Build history of the part. All positions in model axes, mm. A direction names the side the tool comes from. Coordinates: 2 decimals unless noted, no trailing zeros. Order: outer loops, then holes, each group sorted by start corner. A loop starts at its lowest first (then second) coordinate and runs counter-clockwise, first axis right, second up. Notation, with made-up numbers: (72.5, 27) - (122.5, 27) arc R36 ccw to (122.5, 66) - close; hole circle Ø4 at (50, 35). An arc over 180 degrees is marked (long way). Return JSON: item names as keys, results as strings.
from build123d import *

# Parameters (mm, degrees)
F1_DEPTH = 59.69
F2_DEPTH = 25.4
F4_DEPTH = 7.9375
F6_R     = 6.35


# Not quite as in the source:
# - a feature of the source that left no trace in its solid (it failed there, or was rolled back) is left out


with BuildPart() as f1:
    # F0 (on Front) → F1 (new body, symmetric)
    with BuildSketch(Plane.XZ):
        Polygon((22.225, 9.525), (-41.275, 9.525), (-41.275, -9.525), (41.275, -9.525), (41.275, 9.525), align=None)
    extrude(amount=F1_DEPTH, both=True)

    # F0 (on Front) → F2 (join, symmetric)
    with BuildSketch(Plane.XZ):
        with BuildLine():
            Line((22.225, 27.0002), (22.225, 9.525))
            Line((22.225, 9.525), (41.275, 9.525))
            Line((41.275, 9.525), (41.275, 27.0002))
            ThreePointArc((41.275, 27.0002), (45.9246798487, 38.2255201513), (57.15, 42.8752))
            Line((57.15, 42.8752), (60.325, 42.8752))
            Line((60.325, 42.8752), (60.325, 61.9252))
            Line((60.325, 61.9252), (57.15, 61.9252))
            ThreePointArc((57.15, 61.9252), (32.4542956671, 51.6959043329), (22.225, 27.0002))
        make_face()
        Polygon((85.7749970019, 61.9252), (60.325, 61.9252), (60.325, 42.8752), (85.7749970019, 42.8752), (85.7749970019, 46.5751625597), align=None)
    extrude(amount=F2_DEPTH, both=True)

    # F0 (on Front) → F4 (join, symmetric)
    with BuildSketch(Plane.XZ):
        with BuildLine():
            add(Edge.make_bspline(
                [(-41.275, 9.525), (-41.1301143467, 35.7692055404), (24.3351403624, 62.0320998132), (57.15, 61.9252)],
                knots=[0, 0, 0, 0, 111.5045361635, 111.5045361635, 111.5045361635, 111.5045361635], degree=3))
            Line((-41.275, 9.525), (22.225, 9.525))
            Line((22.225, 9.525), (22.225, 27.0002))
            ThreePointArc((22.225, 27.0002), (32.4542956671, 51.6959043329), (57.15, 61.9252))
        make_face()
    extrude(amount=F4_DEPTH, both=True)

    # F0 (on Front) → F5 (revolve)
    with BuildSketch(Plane.XZ):
        Polygon((85.7749970019, 66.675), (85.7749970019, 61.9252), (85.7749970019, 46.5751625597), (85.7749970019, 42.8752), (85.7749970019, 38.1), (111.125, 38.1), (111.125, 66.675), align=None)
    revolve(axis=Axis((85.7749970019, 0, 56.6250812799), (0, 0, 1)))

    # F6
    f6_edges = [f1.edges().sort_by_distance(p)[0] for p in [
        (41.275, -59.69, 0),
        (-41.275, -59.69, 0),
        (-41.275, 59.69, 0),
        (41.275, 59.69, 0),
    ]]
    fillet(f6_edges, radius=F6_R)


solid = f1.part
1. Probe L1, parallel to Y at x = 48.5, z = 53.5; L2, parallel to Y at x = 19, z = 37; L3, parallel to Z at x = -28, y = -16.5 (3 decimals). List the from-to ranges inside material, lowest first.
Check values:
{"L1": "-25.4 to 25.4", "L2": "-7.94 to 7.94", "L3": "-9.525 to 9.525"}
2. Tool access for faces 1 (the cylindrical face through (32.73, -16.79, 51.97)), 2 (the flat face through (-2, 7.938, 30)), 3 (the flat face through (60, 0, 61.925)), 4 (the flat face through (46, 25.4, 42)): list every direction of +Z, -Z, +X, -X, +Y, -Y with a clear straight run to the whole face (end or side of a thin tool).
Check values:
{"face 1": "+Z, -X, -Y", "face 2": "+Z, -X, +Y", "face 3": "+Z, -X", "face 4": "+Z, +X, -X, +Y"}
3. Drop flat-ended pins along their axis: pin 1 (1.5 mm diameter, centred on x = -23.5, y = -9, fed in from +Z) (3 decimals); pin 2 (8.5 mm diameter, centred on y = -19.5, z = 21, fed in from -X) (3 decimals); pin 3 (10 mm diameter, centred on x = 27.5, z = 51, fed in from -Y). Give the stop position or say it passes through.
Check values:
{"pin 1": "z = 9.525", "pin 2": "x = 22.225", "pin 3": "y = -25.4"}
4. Cut at B-B on x = 87.5. Give the cut face in (y, z) (3 decimals).
Check values:
{"outline": "(-25.291, 38.1) - (25.291, 38.1) - (25.291, 66.675) - (-25.291, 66.675) - close"}
5. Cut at A-A on y = 34.5. Give the cut face in (x, z) (3 decimals), plus the area to 3 significant figures.
Check values:
{"outline": "(-41.275, -9.525) - (41.275, -9.525) - (41.275, 9.525) - (-41.275, 9.525) - close", "area": "1,570 mm²"}
